Here's how the part is built. I have some questions about the finished solid (model axes, mm). Give positions to 0.01 mm unless a question says otherwise; leave off trailing zeros. Loops run counter-clockwise (first coordinate to the right, second up) from the corner with the lowest first, then second, coordinate; pieces in that order, holes last. Notation, with made-up numbers: (-21, 54.25) -> (30, 54.25) arc R13 cw to (30, 70.25) -> close; hole circle Ø10 at (44, 23). An arc over 180 degrees is marked (long way). Answer in a Markdown table with one row per item. Add a question column.
Item 1: For P1, Ø8, axis at x = -19, z = -23, coming from the -Y side; P2, Ø3, axis at y = 3.5, z = -27.5, coming from the -X side, each with a flat end and sliding along its axis, tell me the tip position at first contact or that it passes through.
Item 2: If I drill on line 1 (Z direction, x = -14.5, y = 3.3); line 2 (Z direction, x = -11.5, y = 2.8); line 3 (X direction, y = 0.4, z = -2.5), over which ranges is the centre line in solid material (lowest first)?
Item 3: If we section it at B-B (z = 1.5): Write out the boundary of the cut face in (x, y).
Item 4: If we section it at A-A (x = -22.5): Write out the boundary of the cut face in (y, z).
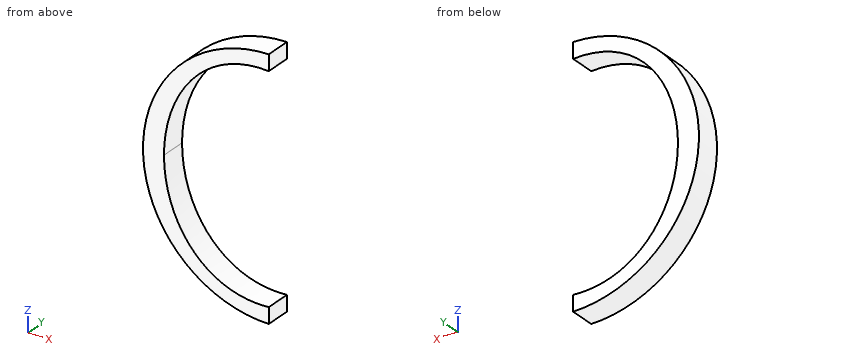
Autodesk Inventor part; units mm, degrees
ref_plane "YZ Plane" through (0, 0, 0) normal (1, 0, 0) x (0, 1, 0)
ref_plane "XZ Plane" through (0, 0, 0) normal (0, 1, 0) x (-1, 0, 0)
ref_plane "XY Plane" through (0, 0, 0) normal (0, 0, 1) x (1, 0, 0)
sketch "Sketch1" plane through (0, 0, 0) normal (0, 1, 0) x (-1, 0, 0)
  line L0 (0, 0) -> (0, -40)
  line L1 (0, -20) -> (20, -20)
  dimension "d0" = 40
  dimension "d1" = 20
sketch "Sketch2" plane through (0, 0, 0) normal (0, 1, 0) x (-1, 0, 0)
  arc A0 (0, -40) -> (0, 0) centre (0, -20) ccw
  line L0 (0, 0) -> (0, 1)
  line L1 (0, -40) -> (0, -41)
  line L2 (0, -20) -> (14.8492, -5.1508) construction
  line L3 (0, -20) -> (0, 1) construction
  spline S0 degree 4 poles (0, 1) (18.89, 2.2775) (28.1468, -20.0014) (18.8898, -42.2749) (0, -41) knots 0 0 0 0 0 1 1 1 1 1
  line L4 (0, 1) -> (0, 4)
  line L5 (0, 4) -> (5, 4)
  line L6 (0, -41) -> (0, -44)
  line L7 (0, -44) -> (5, -44)
  line L8 (20, -20) -> (23, -20)
  arc A1 (24, -20) -> (0, 4) centre (0, -20) ccw
  arc A2 (0, -44) -> (24, -20) centre (0, -20) ccw
  point P0 (14.8493, -34.8486)
  dimension "d4" = 1
  dimension "d5" = 1
  dimension "d6" = 45
  dimension "d7" = 3
  dimension "d8" = 5
  dimension "d9" = 3
  dimension "d10" = 5
  dimension "d11" = 3
extrude "Extrusion1" add sketch "Sketch2" along normal blind 5 contours S0 L4 A1 A2 L6
properties part number "BassGuitarCurveTest"
Recorded:
| question | item | result |
|---|---|---|
| 1 | P1 | stops at y = 0 |
| 1 | P2 | stops at x = -23.24 |
| 2 | line 1 | z = -39.12 to -35.25, -4.75 to -0.88 |
| 2 | line 2 | z = -41.07 to -37.92, -2.08 to 1.07 |
| 2 | line 3 | x = -16.42 to -12.07 |
| 3 | outline | (-10.67, 0) -> (0, 0) -> (0, 5) -> (-10.67, 5) -> close |
| 4 | outline | (0, -28.35) -> (5, -28.35) -> (5, -11.65) -> (0, -11.65) -> close |
